```python
from build123d import *

# Parameters (mm, degrees)
F0_R     = 2.54
F1_DEPTH = 1.27
F2_R     = 2.54
F2_R_2   = 1.524
F3_DEPTH = 13.97
F4_SIZE2 = 4.3215167465
F4_SIZE  = 0.762


with BuildPart() as f1:
    # F0 (on Top) → F1 (new body)
    with BuildSketch(Plane.XY):
        Circle(F0_R)
    extrude(amount=F1_DEPTH)

    # F2 (on face) → F3 (join)
    with BuildSketch(Plane.XY.offset(1.27)):
        Circle(F2_R)
        Circle(F2_R_2, mode=Mode.SUBTRACT)
    extrude(amount=F3_DEPTH)

    # F4
    f4_edges = [f1.edges().sort_by_distance(p)[0] for p in [
        (-2.54, 0, 15.24),
    ]]
    f4_side = f1.faces().sort_by_distance((-2.468158, 0, 15.24))[0]
    chamfer(f4_edges, length=F4_SIZE, length2=F4_SIZE2, reference=f4_side)


solid = f1.part
```
CAD build for the part. Positions are in the model's coordinates, mm. A direction names the side the tool comes from. Round coordinates to 2 decimals unless told otherwise and drop trailing zeros. Order: outer loops, then holes, each group sorted by start corner. A loop starts at its lowest first (then second) coordinate and runs counter-clockwise, first axis right, second up. Notation, with made-up numbers: (27.5, 48) - (79.5, 48) arc R30 cw to (79.5, 75) - close; hole circle Ø2 at (-16.5, 34). An arc over 180 degrees is marked (long way). Use CSV: the item, a comma, the result in double quotes. Start each with the question number.
1) Tool access for faces 1 (the cylindrical face through (-0.33, 2.52, 5.38)), 2 (the flat face through (0, 0, 1.27)): list every direction of +Z, -Z, +X, -X, +Y, -Y with a clear straight run to the whole face (end or side of a thin tool).
2) Saw through at B-B (z = 6). List the corners of the cut face in (x, y).
3) Wall check: L1, parallel to Y at x = 0, z = 8.5; L2, parallel to X at y = -0.2, z = 11; L3, parallel to Z at x = -1.3, y = -0.4. Give the ranges that are in metal, low to high. Write a range as [from, to].
4) Saw through at D-D (z = 12). List the corners of the cut face in (x, y), and give its area (3 significant figures).
5) Pin check, flat tips, straight feed: pin 1 Ø2 at (y, z) = (2, 13.5) entering from +X; pin 2 Ø1.5 at (x, z) = (-0.5, 4) entering from +Y; pin 3 Ø1 at (x, z) = (-1.5, 9) entering from -Y. Stop position of each tip, or through.
6) Saw through at A-A (y = 0). List the corners of the cut face in (x, z).
7) Two-plate mould, pull along Y, no slides. Class faces 3 (the flat face through (0, 0, 0)), 4 (the cylindrical face through (-0.2, 1.51, 8.16)), 5 (the conical face through (-1.65, -1.265, 13.529)): pulls with the +Y half, pulls with the -Y half, needs draft (parallel to the pull), parting line crosses it, or undercut.
Values follow:
1,face 1,"+Z, -Z"
1,face 2,"+Z"
2,outline,"circle Ø5.08 at (0, 0); hole circle Ø3.05 at (0, 0)"
3,L1,"y = [-2.54, -1.52], [1.52, 2.54]"
3,L2,"x = [-2.52, -1.51], [1.51, 2.52]"
3,L3,"z = [0, 1.27]"
4,outline,"circle Ø4.7 at (0, 0); hole circle Ø3.05 at (0, 0)"
4,area,"10.0 mm2"
5,pin 1,"stops at x = 1.86"
5,pin 2,"stops at y = 2.54"
5,pin 3,"stops at y = -2.33"
6,outline,"(-2.54, 0) - (2.54, 0) - (2.54, 10.92) - (1.78, 15.24) - (1.52, 15.24) - (1.52, 1.27) - (-1.52, 1.27) - (-1.52, 15.24) - (-1.78, 15.24) - (-2.54, 10.92) - close"
7,face 3,"needs draft"
7,face 4,"undercut"
7,face 5,"parting line crosses it"
